Verification items for the finished model (mm, model axes). Face numbers are marked on the shaded views. A direction names the side the tool comes from. Coordinates: 2 decimals unless noted, no trailing zeros. Order: outer loops, then holes, each group sorted by start corner. A loop starts at its lowest first (then second) coordinate and runs counter-clockwise, first axis right, second up. Notation, with made-up numbers: M 21.5,40.5 L 28.5,40.5 A17 cw 28.5,56.5 Z; hole C 40,57 d5. An arc over 180 degrees is marked long. Return JSON: item names as keys, results as strings. Group by question number.
1. Section check C-C, the plane y = 0. Record the cut outline in (x, z).
2. Gauge pin test, flat ends, axial feed: pin 1 (10 mm diameter, centred on y = 4.5, z = 18.5, fed in from -X); pin 2 (6 mm diameter, centred on x = 109.5, z = 11.5, fed in from -Y); pin 3 (12 mm diameter, centred on x = 5.5, y = -13, fed in from +Z). Record the tip position at first contact, or that the pin passes through.
3. Section check D-D, the plane x = 108.5. Record the cut outline in (y, z), plus the area to 3 significant figures.
4. Section check B-B, the plane x = 0. Record the cut outline in (y, z), plus the area to 3 significant figures.
5. Material ranges on line 1 along X through (y, z) = (12, 26); line 2 along Z through (x, y) = (-2.5, 11.5); line 3 along Z through (x, y) = (115, -3), recorded low to high.
6. Set-up check for the marked faces 1, 2, 3 and 4: record each of +Z, -Z, +X, -X, +Y, -Y from which the full face is reachable in a straight line by a thin tool's end or side.
7. Section check A-A, the plane z = 0. Record the cut outline in (x, y).
8. Mould release check, pull along Z, two halves, no side actions. Record for the marked faces 5, 6 and 7: +Z half, -Z half, draft (parallel to the pull), parting line (faces both ways), or undercut.
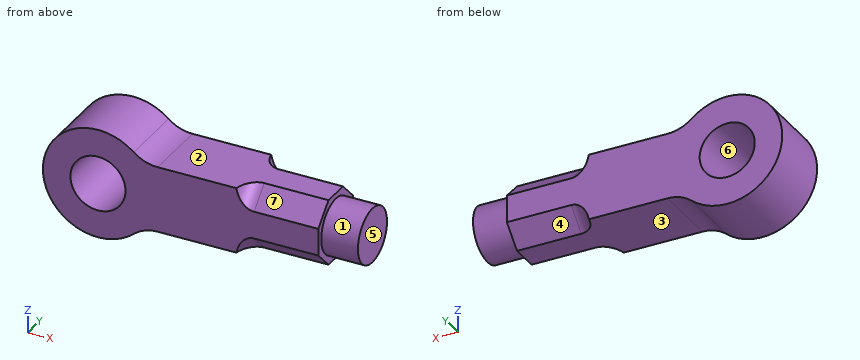
```python
from build123d import *

# Parameters (mm, degrees)
CROQUIS1_R              = 15
SALIENTE_EXTRUIR2_DEPTH = 18
SALIENTE_EXTRUIR3_DEPTH = 45
REDONDEO1_R             = 10
REDONDEO2_R             = 20
CROQUIS3_R              = 15
SALIENTE_EXTRUIR4_DEPTH = 20


with BuildPart() as part:
    # Croquis1 → Saliente-Extruir2 (new, symmetric)
    with BuildSketch(Plane(origin=(0, 0, 0), x_dir=(1, 0, 0), z_dir=(0, 1, 0))):
        with BuildLine():
            Line((24, -18), (75, -18))
            Line((75, -18), (75, 18))
            Line((75, 18), (24, 18))
            ThreePointArc((24, 18), (-30, 0), (24, -18))
        make_face()
        with Locations(Location((0, 0, 0), (0, 0, 270))):
            Circle(CROQUIS1_R, mode=Mode.SUBTRACT)
    extrude(amount=SALIENTE_EXTRUIR2_DEPTH, both=True)

    # Croquis2 → Saliente-Extruir3 (add)
    with BuildSketch(Plane(origin=(75, 0, 0), x_dir=(0, 0, -1), z_dir=(1, 0, 0))):
        Polygon((-18, -7.455844123), (-7.455844123, -18), (7.455844123, -18), (18, -7.455844123), (18, 7.455844123), (7.455844123, 18), (-7.455844123, 18), (-18, 7.455844123), align=None)
    extrude(amount=SALIENTE_EXTRUIR3_DEPTH)

    # Redondeo1
    # the kernel refuses this fillet: 10 mm, written as the material it adds along each edge
    with BuildSketch(Plane(origin=(75, 10.221825407, 35.67766953), x_dir=(-1.4210854715202005e-15, -0.7071067811865512, 0.7071067811865439), z_dir=(0, -0.7071067811865439, -0.7071067811865512))) as redondeo1_piece_1_section:
        with BuildLine():
            CenterArc((REDONDEO1_R, -REDONDEO1_R), REDONDEO1_R, 90, 90)
            Line((0, -REDONDEO1_R), (0, 0))
            Line((0, 0), (REDONDEO1_R, 0))
        make_face()
    redondeo1_piece_1 = extrude(amount=64.911688245, mode=Mode.PRIVATE)
    redondeo1_piece_1 = split(redondeo1_piece_1, bisect_by=Plane(origin=(77.775136413, -18, 13.729156697), z_dir=(0, 1, 0)), keep=Keep.TOP, mode=Mode.PRIVATE)
    redondeo1_piece_1 = split(redondeo1_piece_1, bisect_by=Plane(origin=(77.775136413, -13.729156697, 18), z_dir=(0, 0, -1)), keep=Keep.TOP, mode=Mode.PRIVATE)
    add(redondeo1_piece_1)
    with BuildSketch(Plane(origin=(75, -35.67766953, 10.221825407), x_dir=(0, -0.707106781186544, -0.7071067811865511), z_dir=(0, 0.7071067811865511, -0.7071067811865441))) as redondeo1_piece_2_section:
        with BuildLine():
            CenterArc((REDONDEO1_R, -REDONDEO1_R), REDONDEO1_R, 90, 90)
            Line((0, -REDONDEO1_R), (0, 0))
            Line((0, 0), (REDONDEO1_R, 0))
        make_face()
    redondeo1_piece_2 = extrude(amount=64.911688245, mode=Mode.PRIVATE)
    redondeo1_piece_2 = split(redondeo1_piece_2, bisect_by=Plane(origin=(77.775136413, -18, -13.729156697), z_dir=(0, 1, 0)), keep=Keep.TOP, mode=Mode.PRIVATE)
    redondeo1_piece_2 = split(redondeo1_piece_2, bisect_by=Plane(origin=(77.775136413, -13.729156697, -18), z_dir=(0, 0, 1)), keep=Keep.TOP, mode=Mode.PRIVATE)
    add(redondeo1_piece_2)
    with BuildSketch(Plane(origin=(75, -10.221825407, -35.67766953), x_dir=(1.421085471520201e-15, 0.7071067811865511, -0.7071067811865439), z_dir=(0, 0.7071067811865439, 0.7071067811865511))) as redondeo1_piece_3_section:
        with BuildLine():
            CenterArc((REDONDEO1_R, -REDONDEO1_R), REDONDEO1_R, 90, 90)
            Line((0, -REDONDEO1_R), (0, 0))
            Line((0, 0), (REDONDEO1_R, 0))
        make_face()
    redondeo1_piece_3 = extrude(amount=64.911688245, mode=Mode.PRIVATE)
    redondeo1_piece_3 = split(redondeo1_piece_3, bisect_by=Plane(origin=(77.775136413, 18, -13.729156697), z_dir=(0, -1, 0)), keep=Keep.TOP, mode=Mode.PRIVATE)
    redondeo1_piece_3 = split(redondeo1_piece_3, bisect_by=Plane(origin=(77.775136413, 13.729156697, -18), z_dir=(0, 0, 1)), keep=Keep.TOP, mode=Mode.PRIVATE)
    add(redondeo1_piece_3)
    with BuildSketch(Plane(origin=(75, 35.67766953, -10.221825407), x_dir=(0, 0.7071067811865458, 0.7071067811865493), z_dir=(0, -0.7071067811865493, 0.7071067811865458))) as redondeo1_piece_4_section:
        with BuildLine():
            CenterArc((REDONDEO1_R, -REDONDEO1_R), REDONDEO1_R, 90, 90)
            Line((0, -REDONDEO1_R), (0, 0))
            Line((0, 0), (REDONDEO1_R, 0))
        make_face()
    redondeo1_piece_4 = extrude(amount=64.911688245, mode=Mode.PRIVATE)
    redondeo1_piece_4 = split(redondeo1_piece_4, bisect_by=Plane(origin=(77.775136413, 13.729156697, 18), z_dir=(0, 0, -1)), keep=Keep.TOP, mode=Mode.PRIVATE)
    redondeo1_piece_4 = split(redondeo1_piece_4, bisect_by=Plane(origin=(77.775136413, 18, 13.729156697), z_dir=(0, -1, 0)), keep=Keep.TOP, mode=Mode.PRIVATE)
    add(redondeo1_piece_4)

    # Redondeo2
    redondeo2_edges = [part.edges().sort_by_distance(p)[0] for p in [
        (24, 0, 18),
        (24, 0, -18),
    ]]
    fillet(redondeo2_edges, radius=REDONDEO2_R)

    # Croquis3 → Saliente-Extruir4 (add)
    with BuildSketch(Plane(origin=(120, 0, 0), x_dir=(0, 0, -1), z_dir=(1, 0, 0))):
        with Locations(Location((0, 0, 0), (0, 0, 90))):
            Circle(CROQUIS3_R)
    extrude(amount=SALIENTE_EXTRUIR4_DEPTH)


solid = part.part
```
Answers follow:
{
 "1": {"outline": "M 19.5,-22.8 A20 cw 32.5,-18 L 120,-18 L 120,-15 L 140,-15 L 140,15 L 120,15 L 120,18 L 32.5,18 A20 cw 19.5,22.8 A30 ccw long Z; hole C 0,0 d30"},
 "2": {"pin 1": "x = -26.79", "pin 2": "y = -16.96", "pin 3": "z = 30"},
 "3": {"outline": "M -18,-7.46 L -7.46,-18 L 7.46,-18 L 18,-7.46 L 18,7.46 L 7.46,18 L -7.46,18 L -18,7.46 Z", "area": "1,070 mm^2"},
 "4": {"outline": "M -18,-30 L 18,-30 L 18,-15 L -18,-15 Z; M -18,15 L 18,15 L 18,30 L -18,30 Z", "area": "1,080 mm^2"},
 "5": {"line 1": "-14.97 to 14.97", "line 2": "-29.9 to -14.79, 14.79 to 29.9", "line 3": "-18 to 18"},
 "6": {"face 1": "+X", "face 2": "+Z, +X, +Y, -Y", "face 3": "-Z, +X, +Y, -Y", "face 4": "-Z, +X, +Y"},
 "7": {"outline": "M -30,-18 L -15,-18 L -15,18 L -30,18 Z; M 15,-18 L 120,-18 L 120,-15 L 140,-15 L 140,15 L 120,15 L 120,18 L 15,18 Z"},
 "8": {"face 5": "draft", "face 6": "undercut", "face 7": "+Z half"}
}
